from build123d import *

# Parameters (mm, degrees)
SKETCH2_W           = 203.2
SKETCH2_H           = 127
BOSS_EXTRUDE2_DEPTH = 17.78
FILLET1_R           = 12.7
SKETCH5_R           = 2.0828
CUT_EXTRUDE2_DEPTH  = 12.7


with BuildPart() as part:
    # Sketch2 → Boss-Extrude2 (new body)
    with BuildSketch(Plane(origin=(0, 0, 0), x_dir=(1, 0, 0), z_dir=(0, 1, 0))):
        Rectangle(SKETCH2_W, SKETCH2_H)
    extrude(amount=BOSS_EXTRUDE2_DEPTH)

    # Fillet1
    fillet1_edges = [part.edges().sort_by_distance(p)[0] for p in [
        (-101.6, 8.89, -63.5),
        (101.6, 8.89, -63.5),
    ]]
    fillet(fillet1_edges, radius=FILLET1_R)

    # Sketch5 → Cut-Extrude2 (cut)
    with BuildSketch(Plane.XZ):
        with Locations(Location((50.8, 49.8348, 0), (0, 0, 270))):
            Circle(SKETCH5_R)
        with Locations(Location((33.5788, 25.0698, 0), (0, 0, 270))):
            Circle(SKETCH5_R)
        with Locations(Location((-50.8, 25.0698, 0), (0, 0, 270))):
            Circle(SKETCH5_R)
        with Locations(Location((-33.5788, 49.8348, 0), (0, 0, 270))):
            Circle(SKETCH5_R)
    extrude(amount=-CUT_EXTRUDE2_DEPTH, mode=Mode.SUBTRACT)


solid = part.part
Here's how the part is built. I have some questions about the finished solid (model axes, mm). A direction names the side the tool comes from. Round coordinates to 2 decimals unless told otherwise and drop trailing zeros. Loops run counter-clockwise (first coordinate to the right, second up) from the corner with the lowest first, then second, coordinate; pieces in that order, holes last. Notation, with made-up numbers: (1.5, 17.5) - (31.5, 17.5) arc R21 cw to (31.5, 54.5) - close; hole circle Ø8 at (37, 9.25). An arc over 180 degrees is marked (long way). One line per question, with ' | ' between items. Start each with the question number.
Q1. For faces 1 (the cylindrical face through (-32.95, 6.26, 47.85)), 2 (the flat face through (-1, 9, -63.5)), which set-ups out of +Z, -Z, +X, -X, +Y, -Y let a thin tool reach every point of the face, with its end or its side?
Q2. Please list where these lines run through material, in increasing order: line 1 (Z direction, x = 89.5, y = 12); line 2 (Z direction, x = -33, y = 1). Write a range as [from, to].
Q3. Will these pins go through, and if not, where does the flat tip stop? pin 1 (4.5 mm diameter, centred on x = -51.5, z = 25, fed in from -Y); pin 2 (1.2 mm diameter, centred on x = -33, z = 50, fed in from -Y).
Q4. I want a section at A-A (x = 50.8). Write out the boundary of the cut face in (y, z), then the cut area to 3 significant figures.
Response values:
1) face 1: -Y | face 2: -Z, +X, -X, +Y, -Y
2) line 1: z = [-63.49, 63.5] | line 2: z = [-63.5, 47.83], [51.84, 63.5]
3) pin 1: stops at y = 0 | pin 2: stops at y = 12.7
4) outline: (0, -63.5) - (17.78, -63.5) - (17.78, 63.5) - (0, 63.5) - (0, 51.92) - (12.7, 51.92) - (12.7, 47.75) - (0, 47.75) - close | area: 2,210 mm²
